The model under review builds one solid part; all positions refer to its coordinate system, in mm. A direction names the side the tool comes from. Give positions to 0.01 mm unless a question says otherwise; leave off trailing zeros. Write each loop counter-clockwise with the first axis right and the second up, starting at its lowest first coordinate (ties: lowest second). Pieces come first, ordered by that corner, then holes. Notation, with made-up numbers: (-17, 39.25) -> (7, 39.25) arc R11 ccw to (7, 55.25) -> close; hole circle Ø4 at (-33, -35.75). An arc over 180 degrees is marked (long way). Use CSV: the item, a comma, the result in double quotes.
```python
from build123d import *
from build123d.topology import SkipClean

# Parameters (mm, degrees)
SKETCH_5_W                 = 18
SKETCH_5_H                 = 100
EXTRUDE_1_DEPTH            = 15
PATTERN_LINEAR_1_COUNT     = 2
PATTERN_LINEAR_1_PITCH     = 16.1
PATTERN_LINEAR_1_COL_COUNT = 2
PATTERN_LINEAR_1_COL_PITCH = 16.1
SKETCH_9_W                 = 55
SKETCH_9_H                 = 5
CUT_EXTRUDE_1_DEPTH        = 109.050913925
CUT_EXTRUDE_1_DEPTH_BACK   = 109.050913925
SKETCH_12_R                = 3.25
SKETCH_15_R                = 8
CUT_EXTRUDE_4_DEPTH        = 109.050913925
SKETCH_17_W                = 8.2
SKETCH_17_H                = 55
SKETCH_19_R                = 1.75
CUT_EXTRUDE_7_DEPTH        = 109.050913925
PATTERN_LINEAR_2_COUNT     = 3
PATTERN_LINEAR_2_PITCH     = 16.4
MIRROR_7_COPY_1_SKETCH_R   = 1.75
MIRROR_7_COPY_1_DEPTH      = 109.050913925
MIRROR_7_COPY_2_SKETCH_R   = 1.75
MIRROR_7_COPY_2_DEPTH      = 109.050913925


with BuildPart() as part:
    # Sketch 5 → Extrude 1 (new, symmetric)
    with BuildSketch(Plane.XY):
        with Locations((-9, 20)):
            Rectangle(SKETCH_5_W, SKETCH_5_H)
    extrude_1 = extrude(amount=EXTRUDE_1_DEPTH, both=True)

    # Sketch 7 → Cut-Revolve 1 (revolve, cut)
    with BuildSketch(Plane.XY):
        with BuildLine():
            Line((-18, 8), (-18, -8))
            ThreePointArc((-18, -8), (-10, 0), (-18, 8))
        make_face()
    cut_revolve_1 = revolve(axis=Axis((-18, 8, 0), (0, -1, 0)), mode=Mode.SUBTRACT)

    # Pattern Linear 1: Cut-Revolve 1 ×2
    with Locations(*[(0, i * PATTERN_LINEAR_1_PITCH, 0) for i in range(1, PATTERN_LINEAR_1_COUNT)]):
        add(cut_revolve_1, mode=Mode.SUBTRACT)

    # Pattern Linear 1 col: Cut-Revolve 1 ×2
    with Locations(*[(0, -i * PATTERN_LINEAR_1_COL_PITCH, 0) for i in range(1, PATTERN_LINEAR_1_COL_COUNT)]):
        add(cut_revolve_1, mode=Mode.SUBTRACT)

    # Mirror 2: Extrude 1 across plane
    add(extrude_1.mirror(Plane(origin=(0, 0, 0), x_dir=(0, 0, 1), z_dir=(1, 0, 0))))

    # Mirror 3: Cut-Revolve 1 across plane
    with SkipClean():  # the faces are left unmerged after this step: merging them gives an invalid solid
        add(cut_revolve_1.mirror(Plane(origin=(0, 0, 0), x_dir=(0, 0, 1), z_dir=(1, 0, 0))), mode=Mode.SUBTRACT)

    # Mirror 4 copy 1 sketch → Mirror 4 copy 1 (revolve, cut)
    with SkipClean():  # the faces are left unmerged after this step: merging them gives an invalid solid
        with BuildSketch(Plane(origin=(0, 16.1, 0), x_dir=(-1, 0, 0), z_dir=(0, 0, 1))):
            with BuildLine():
                Line((-18, -8), (-18, 8))
                ThreePointArc((-18, 8), (-10, 0), (-18, -8))
            make_face()
        revolve(axis=Axis((18, 24.1, 0), (0, 1, 0)), mode=Mode.SUBTRACT)

    # Mirror 4 copy 2 sketch → Mirror 4 copy 2 (revolve, cut)
    with SkipClean():  # the faces are left unmerged after this step: merging them gives an invalid solid
        with BuildSketch(Plane(origin=(0, -16.1, 0), x_dir=(-1, 0, 0), z_dir=(0, 0, 1))):
            with BuildLine():
                Line((-18, -8), (-18, 8))
                ThreePointArc((-18, 8), (-10, 0), (-18, -8))
            make_face()
        revolve(axis=Axis((18, -8.1, 0), (0, 1, 0)), mode=Mode.SUBTRACT)

    # Mirror 4 copy 3 sketch → Mirror 4 copy 3 (revolve, cut)
    with SkipClean():  # the faces are left unmerged after this step: merging them gives an invalid solid
        with BuildSketch(Plane(origin=(0, 0, 0), x_dir=(-1, 0, 0), z_dir=(0, 0, 1))):
            with BuildLine():
                Line((-18, -8), (-18, 8))
                ThreePointArc((-18, 8), (-10, 0), (-18, -8))
            make_face()
        revolve(axis=Axis((18, 8, 0), (0, 1, 0)), mode=Mode.SUBTRACT)

    # Sketch 9 → Revolve 1 (revolve)
    with SkipClean():  # the faces are left unmerged after this step: merging them gives an invalid solid
        with BuildSketch(Plane.XY, mode=Mode.PRIVATE) as revolve_1_sk:
            with Locations((27.5, 72.5)):
                Rectangle(SKETCH_9_W, SKETCH_9_H)
        revolve(revolve_1_sk.sketch.rotate(Axis((0, 70, 0), (0, 1, 0)), 90), axis=Axis((0, 70, 0), (0, 1, 0)))

    # Sketch 12 → Cut-Extrude 1 (cut, two sides: drawn at the far end of the back side and taken through both)
    with SkipClean():  # the faces are left unmerged after this step: merging them gives an invalid solid
        with BuildSketch(Plane(origin=(0, 0, 0), x_dir=(1, 0, 0), z_dir=(0, 1, 0)).offset(-CUT_EXTRUDE_1_DEPTH_BACK)):
            with Locations(Location((0, 0, 0), (0, 0, 270))):
                Circle(SKETCH_12_R)
        extrude(amount=CUT_EXTRUDE_1_DEPTH + CUT_EXTRUDE_1_DEPTH_BACK, mode=Mode.SUBTRACT)

    # Sketch 15 → Cut-Extrude 4 (cut, through all)
    with SkipClean():  # the faces are left unmerged after this step: merging them gives an invalid solid
        with BuildSketch(Plane(origin=(0, 0, 0), x_dir=(1, 0, 0), z_dir=(0, 1, 0))):
            with Locations(Location((0, 0, 0), (0, 0, 270))):
                Circle(SKETCH_15_R)
        extrude(amount=-CUT_EXTRUDE_4_DEPTH, mode=Mode.SUBTRACT)

    # Sketch 18 → Cut-Revolve 2 (revolve, cut)
    with SkipClean():  # the faces are left unmerged after this step: merging them gives an invalid solid
        with BuildSketch(Plane.XY):
            with BuildLine():
                Line((-18, 33.2), (-18, 16.8))
                ThreePointArc((-18, 16.8), (-9.8, 25), (-18, 33.2))
            make_face()
        cut_revolve_2 = revolve(axis=Axis((-18, 33.2, 0), (0, -1, 0)), mode=Mode.SUBTRACT)

    # Sketch 17 → Cut-Revolve 3 (revolve, cut)
    with SkipClean():  # the faces are left unmerged after this step: merging them gives an invalid solid
        with BuildSketch(Plane.XY):
            with Locations((-13.9, -2.5)):
                Rectangle(SKETCH_17_W, SKETCH_17_H)
        cut_revolve_3 = revolve(axis=Axis((-18, -30, 0), (0, 1, 0)), mode=Mode.SUBTRACT)

    # Mirror 5: Cut-Revolve 2 across plane
    with SkipClean():  # the faces are left unmerged after this step: merging them gives an invalid solid
        add(cut_revolve_2.mirror(Plane(origin=(0, 0, 0), x_dir=(0, 0, 1), z_dir=(1, 0, 0))), mode=Mode.SUBTRACT)

    # Mirror 6: Cut-Revolve 3 across plane
    with SkipClean():  # the faces are left unmerged after this step: merging them gives an invalid solid
        add(cut_revolve_3.mirror(Plane(origin=(0, 0, 0), x_dir=(0, 0, 1), z_dir=(1, 0, 0))), mode=Mode.SUBTRACT)

    # Sketch 19 → Cut-Extrude 7 (cut, symmetric)
    with SkipClean():  # the faces are left unmerged after this step: merging them gives an invalid solid
        with BuildSketch(Plane.XY):
            with Locations((-15, 16.2)):
                Circle(SKETCH_19_R)
        cut_extrude_7 = extrude(amount=CUT_EXTRUDE_7_DEPTH, both=True, mode=Mode.SUBTRACT)

    # Pattern Linear 2: Cut-Extrude 7 ×3
    with SkipClean():  # the faces are left unmerged after this step: merging them gives an invalid solid
        with Locations(*[(0, -i * PATTERN_LINEAR_2_PITCH, 0) for i in range(1, PATTERN_LINEAR_2_COUNT)]):
            add(cut_extrude_7, mode=Mode.SUBTRACT)

    # Mirror 7: Cut-Extrude 7 across plane
    with SkipClean():  # the faces are left unmerged after this step: merging them gives an invalid solid
        add(cut_extrude_7.mirror(Plane(origin=(0, 0, 0), x_dir=(0, 0, 1), z_dir=(1, 0, 0))), mode=Mode.SUBTRACT)

    # Mirror 7 copy 1 sketch → Mirror 7 copy 1 (cut, symmetric)
    with SkipClean():  # the faces are left unmerged after this step: merging them gives an invalid solid
        with BuildSketch(Plane(origin=(0, -16.4, 0), x_dir=(-1, 0, 0), z_dir=(0, 0, 1))):
            with Locations((-15, -16.2)):
                Circle(MIRROR_7_COPY_1_SKETCH_R)
        extrude(amount=MIRROR_7_COPY_1_DEPTH, both=True, mode=Mode.SUBTRACT)

    # Mirror 7 copy 2 sketch → Mirror 7 copy 2 (cut, symmetric)
    with SkipClean():  # the faces are left unmerged after this step: merging them gives an invalid solid
        with BuildSketch(Plane(origin=(0, -32.8, 0), x_dir=(-1, 0, 0), z_dir=(0, 0, 1))):
            with Locations((-15, -16.2)):
                Circle(MIRROR_7_COPY_2_SKETCH_R)
        extrude(amount=MIRROR_7_COPY_2_DEPTH, both=True, mode=Mode.SUBTRACT)


solid = part.part
```
Q1. Insertion check: pin 1 (8 mm diameter, centred on x = -42.5, z = 30.5, fed in from -Y); pin 2 (1 mm diameter, centred on x = -14, y = 14, fed in from -Z); pin 3 (5.5 mm diameter, centred on x = -15, y = -0.2, fed in from +Z); pin 4 (5 mm diameter, centred on x = 0, z = 0, fed in from +Y). Each pin has a flat end and moves straight along its axis. Give the tip position at first contact, or say it passes through.
Derived:
pin 1,"stops at y = 70"
pin 2,"stops at z = -15"
pin 3,"stops at z = 15"
pin 4,"passes through"
Q2. The part is to be moulded in two halves that separate along Z. For faces 6 (the flat face through (0, 21, -15)), 7 (the flat face through (0.1, 0, 3.4)), 8 (the cylindrical face through (13.383, 15.53, -11.708)), say which applies: pulls with the +Z half, pulls with the -Z half, needs draft (parallel to the pull), parting line crosses it, or undercut.
Derived:
face 6,"pulls with the -Z half"
face 7,"undercut"
face 8,"needs draft"
Q3. Consider section D-D (z = -10.5). Write out the cut boundary in (x, y), then the cut area to 3 significant figures.
Derived:
outline,"(-53.99, 70) -> (-18, 70) -> (-18, -30) -> (18, -30) -> (18, 70) -> (53.99, 70) -> (53.99, 75) -> (-53.99, 75) -> close; hole circle Ø3.5 at (-15, -16.6); hole circle Ø3.5 at (-15, -0.2); hole circle Ø3.5 at (-15, 16.2); hole circle Ø3.5 at (15, -16.6); hole circle Ø3.5 at (15, -0.2); hole circle Ø3.5 at (15, 16.2)"
area,"4,080 mm2"
Q4. Consider section A-A (x = 0). Write out the cut boundary in (y, z), then the cut area to 3 significant figures.
Derived:
outline,"(-30, -15) -> (70, -15) -> (70, -55) -> (75, -55) -> (75, -3.25) -> (0, -3.25) -> (0, -8) -> (-30, -8) -> close; (-30, 8) -> (0, 8) -> (0, 3.25) -> (75, 3.25) -> (75, 55) -> (70, 55) -> (70, 15) -> (-30, 15) -> close"
area,"2,580 mm2"
Q5. To check wall thickness, follow probe 1 along Y at (x, z) = (15, -10); probe 2 along Z at (x, y) = (0, 23); probe 3 along Z at (x, y) = (-7, 34.5). State the ranges of each line that lie inside material, in increasing order.
Derived:
probe 1,"y = -30 to -18.35, -14.85 to -1.95, 1.55 to 14.45, 17.95 to 75"
probe 2,"z = -15 to -3.25, 3.25 to 15"
probe 3,"z = -15 to 15"
Q6. Machinability: for faces 1 (the flat face through (18, 30, 7)), 2 (the flat face through (0, 21, 15)), 3 (the flat face through (-18, 30, 7)), 4 (the cylindrical face through (-7.81, -14.79, -1.73)), 5 (the flat face through (11, 75, -1)), which of the approach directions +Z, -Z, +X, -X, +Y, -Y give a long, thin tool a straight path to every point of the face, cutting with its end or side? Answer none if there is none.
Derived:
face 1,"+Z, -Z, +X, -Y"
face 2,"+Z, +X, -X, -Y"
face 3,"+Z, -Z, -X, -Y"
face 4,"-Y"
face 5,"+Z, -Z, +X, -X, +Y"
Q7. Consider section B-B (y = -16.6). Write out the cut boundary in (x, z).
Derived:
outline,"(-18, -15) -> (-16.75, -15) -> (-16.75, -8.1) arc R8.2 cw to (-18, -8.2) -> close; (-18, 8.2) arc R8.2 cw to (-16.75, 8.1) -> (-16.75, 15) -> (-18, 15) -> close; (-13.25, -15) -> (13.25, -15) -> (13.25, -6.68) arc R8.2 cw to (13.25, 6.68) -> (13.25, 15) -> (-13.25, 15) -> (-13.25, 6.68) arc R8.2 cw to (-13.25, -6.68) -> close; (16.75, -15) -> (18, -15) -> (18, -8.2) arc R8.2 cw to (16.75, -8.1) -> close; (16.75, 8.1) arc R8.2 cw to (18, 8.2) -> (18, 15) -> (16.75, 15) -> close; hole circle Ø16 at (0, 0)"
Q8. Consider section C-C (y = 51.5). Write out the cut boundary in (x, z), then the cut area to 3 significant figures.
Derived:
outline,"(-18, -15) -> (18, -15) -> (18, 15) -> (-18, 15) -> close; hole circle Ø6.5 at (0, 0)"
area,"1,050 mm2"
